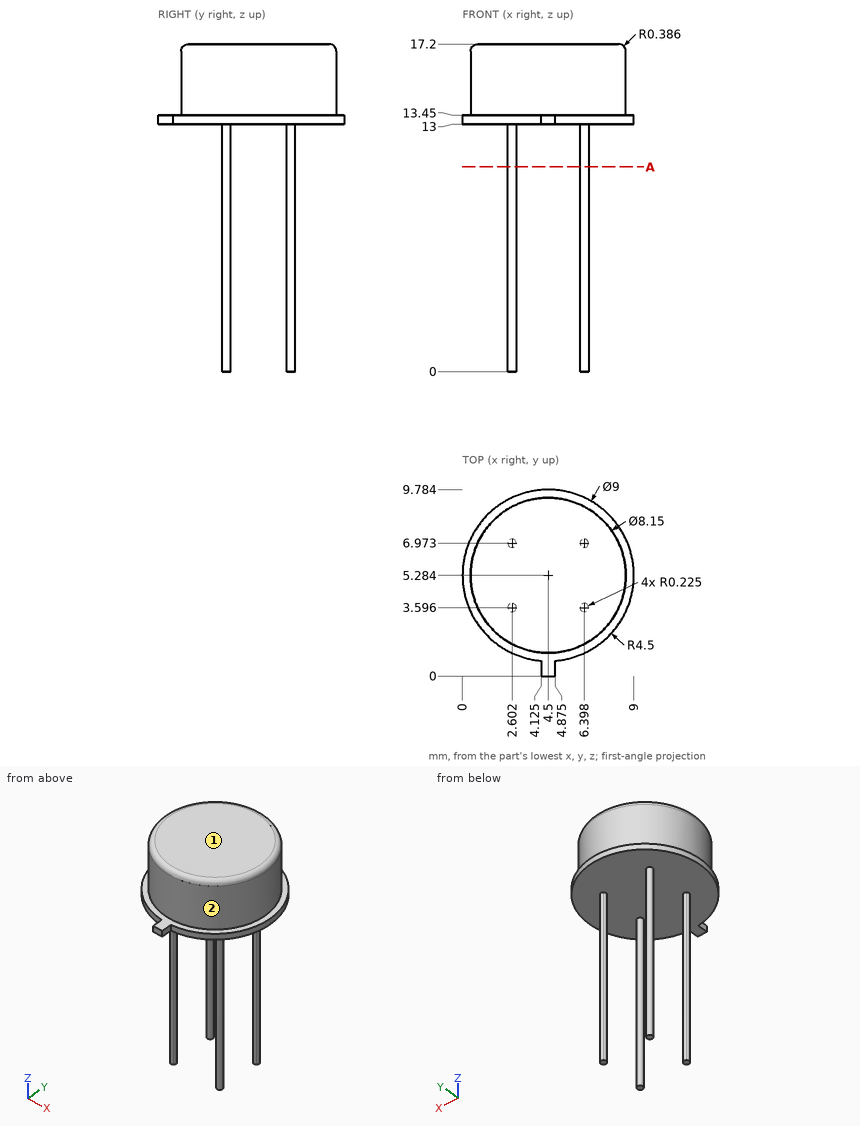
Geometry check sheet. Reference: drawing and pictorial views, mm from the part's lowest x, y, z. A direction names the side the tool comes from. Round coordinates to 2 decimals unless told otherwise and drop trailing zeros. Answer as CSV lines item,"result". Start each with the question number.
1) Tool access check on the marked faces 1 and 2. Record the directions out of +Z, -Z, +X, -X, +Y, -Y that give a thin tool (end or side, any length) a straight path to the whole face; none if there is none.
2) Material ranges on line 1 (Z direction, x = 3.25, y = 5.5); line 2 (X direction, y = 3.5, z = 12.5) (1 decimal); line 3 (Y direction, x = 6.5, z = 13.75) (1 decimal), recorded low to high. Write a range as from..to.
3) Go/stop test with flat-tipped pins: P1, Ø5, axis at y = 5, z = 4.5, coming from the +X side; P2, Ø2.5, axis at x = 5, y = 4.5, coming from the -Z side. Record where each tip stops, or that it passes through.
4) Section check A-A on z = 10.75. State how many separate pieces and enclosed holes the cut face has.
Found:
1,face 1,"+Z, +X, -X, +Y, -Y"
1,face 2,"+Z"
2,line 1,"z = 13..17.2"
2,line 2,"x = 2.4..2.8, 6.2..6.6"
2,line 3,"y = 1.7..8.8"
3,P1,"stops at x = 6.62"
3,P2,"stops at z = 13"
4,separate pieces,"4"
4,enclosed holes,"0"
